from build123d import *

# Parameters (mm, degrees)
BOSS_EXTRUDE1_DEPTH = 12.7
CUT_EXTRUDE1_START  = 12.7
SKETCH2_R           = 2.38125
CUT_EXTRUDE1_DEPTH  = 13.7


with BuildPart() as part:
    # Sketch1 → Boss-Extrude1 (new body)
    with BuildSketch(Plane(origin=(0, 0, 0), x_dir=(1, 0, 0), z_dir=(0, 1, 0))):
        with BuildLine():
            Line((-73.025, 50.8), (73.025, 50.8))
            ThreePointArc((73.025, 50.8), (75.27006403, 49.87006403), (76.2, 47.625))
            Line((76.2, 47.625), (76.2, -47.625))
            ThreePointArc((76.2, -47.625), (75.27006403, -49.87006403), (73.025, -50.8))
            Line((73.025, -50.8), (-73.025, -50.8))
            ThreePointArc((-73.025, -50.8), (-75.27006403, -49.87006403), (-76.2, -47.625))
            Line((-76.2, -47.625), (-76.2, 47.625))
            ThreePointArc((-76.2, 47.625), (-75.27006403, 49.87006403), (-73.025, 50.8))
        make_face()
    extrude(amount=BOSS_EXTRUDE1_DEPTH)

    # Sketch2 → Cut-Extrude1 (cut, through all)
    with BuildSketch(Plane(origin=(0, 0, 0), x_dir=(1, 0, 0), z_dir=(0, 1, 0)).offset(CUT_EXTRUDE1_START)):
        Circle(SKETCH2_R)
    extrude(amount=-CUT_EXTRUDE1_DEPTH, mode=Mode.SUBTRACT)


solid = part.part
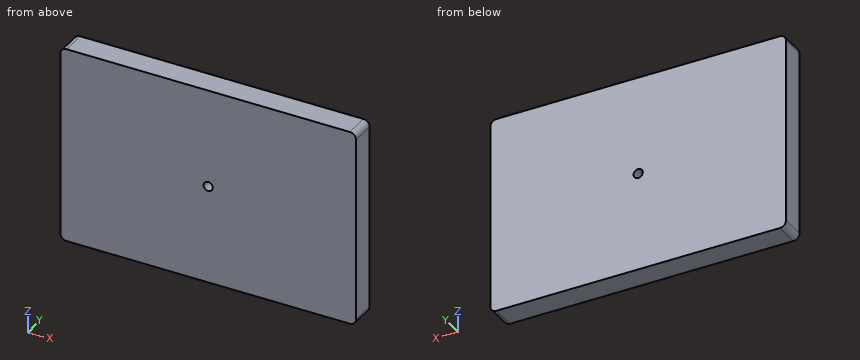
Work out the finished part from the listing and answer in its coordinate system (mm). Round coordinates to 2 decimals unless told otherwise and drop trailing zeros. Loops run counter-clockwise (first coordinate to the right, second up) from the corner with the lowest first, then second, coordinate; pieces in that order, holes last. Notation, with made-up numbers: (10, -6.75) -> (22, -6.75) arc R11 cw to (22, 3.25) -> close; hole circle Ø10 at (-0.5, 81). An arc over 180 degrees is marked (long way). Use one line per item in the form item = value.
(1) Find section A-A on z = 0. Give the vertices of the cut face in (x, y).
Answer list:
outline = (-76.2, 0) -> (-2.38, 0) -> (-2.38, 12.7) -> (-76.2, 12.7) -> close; (2.38, 0) -> (76.2, 0) -> (76.2, 12.7) -> (2.38, 12.7) -> close
(2) Straight lines are drawn through the part: line 1 (Z direction, x = 0, y = 9.75); line 2 (X direction, y = 5.75, z = 0). For each, find the intervals that lie inside material, in ascending order.
Answer list:
line_1 = -50.8 to -2.38, 2.38 to 50.8
line_2 = -76.2 to -2.38, 2.38 to 76.2
(3) Find section B-B on x = 0. Give the vertices of the cut face in (y, z), then the cut area to 3 significant figures.
Answer list:
outline = (0, -50.8) -> (12.7, -50.8) -> (12.7, -2.38) -> (0, -2.38) -> close; (0, 2.38) -> (12.7, 2.38) -> (12.7, 50.8) -> (0, 50.8) -> close
area = 1,230 mm2
